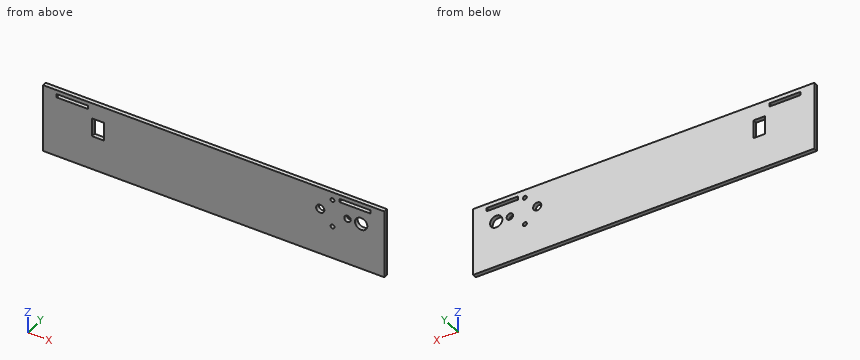
```python
from build123d import *

# Parameters (mm, degrees)
F0_W     = 250
F0_H     = 50
F1_DEPTH = 3
F2_DEPTH = 3
F3_R     = 4.5
F3_R_2   = 1.45
F3_R_3   = 2.375
F3_R_4   = 3
F3_W     = 8.5
F3_H     = 13.5
F4_DEPTH = 25


# Not quite as in the source:
# - ends of sketch curves that miss each other by under 0.0002 mm in the source are joined


with BuildPart() as f1:
    # F0 (on Front) → F1 (new body)
    with BuildSketch(Plane.XZ):
        with Locations((-42.7222467884, 16.2994446903)):
            Rectangle(F0_W, F0_H)
        Polygon((-147.7222467884, 35.7994452119), (-157.7222467884, 35.7994452119), (-157.7222467884, 38.2994446903), (-134.7222467884, 38.2994446903), (-134.7222467884, 35.7994446903), (-144.7222467884, 35.7994446903), align=None, mode=Mode.SUBTRACT)
        Polygon((49.2777532116, 38.2994446903), (62.2777532116, 38.2994446903), (72.2777532116, 38.2994446903), (72.2777532116, 35.7994446903), (49.2777532116, 35.7994446903), align=None, mode=Mode.SUBTRACT)
    extrude(amount=F1_DEPTH)

    # F0 (on Front) → F2 (join)
    with BuildSketch(Plane.XZ):
        with Locations((-42.7222467884, 16.2994446903)):
            Rectangle(F0_W, F0_H)
        Polygon((-147.7222467884, 35.7994452119), (-157.7222467884, 35.7994452119), (-157.7222467884, 38.2994446903), (-134.7222467884, 38.2994446903), (-134.7222467884, 35.7994446903), (-144.7222467884, 35.7994446903), align=None, mode=Mode.SUBTRACT)
        Polygon((49.2777532116, 38.2994446903), (62.2777532116, 38.2994446903), (72.2777532116, 38.2994446903), (72.2777532116, 35.7994446903), (49.2777532116, 35.7994446903), align=None, mode=Mode.SUBTRACT)
    extrude(amount=F2_DEPTH)

    # F3 (on face) → F4 (cut)
    with BuildSketch(Plane(origin=(0, 0, 0), x_dir=(-1, 0, 0), z_dir=(0, 1, 0))):
        with Locations((-65.2777532116, 25.2994446903)):
            Circle(F3_R)
        with Locations((-44.2777532116, 15.2994446903)):
            Circle(F3_R_2)
        with Locations((-44.2777532116, 35.2994446903)):
            Circle(F3_R_2)
        with Locations((-55.2777532116, 25.2994446903)):
            Circle(F3_R_3)
        with Locations((-35.2777532116, 25.2994446903)):
            Circle(F3_R_4)
        with Locations((127.4722467884, 23.0494446903)):
            Rectangle(F3_W, F3_H)
    extrude(amount=-F4_DEPTH, mode=Mode.SUBTRACT)


solid = f1.part
```
CAD build for the part. Positions are in the model's coordinates, mm. Give positions to 0.01 mm unless a question says otherwise; leave off trailing zeros. Write each loop counter-clockwise with the first axis right and the second up, starting at its lowest first coordinate (ties: lowest second). Pieces come first, ordered by that corner, then holes. Notation, with made-up numbers: M 25,6 L 65,6 A20 ccw 65,11 Z; hole C -26,76 d2. An arc over 180 degrees is marked long. Return JSON: item names as keys, results as strings. Group by question number.
(1) Flat gauge pin, fed straight in: pin 1 Ø2.5 at (x, z) = (44.28, 35.3) entering from +Y. Where does the tip first touch, or does it go through?
(2) Drill centre lines: L1, parallel to X at y = -1.6, z = 35; L2, parallel to Z at x = 70, y = -1.25; L3, parallel to X at y = -2.45, z = 17.5. Where is each one in solid material? Low to high. Write a range as [from, to].
(3) Band-saw the part on B-B (y = -2.4). State how many separate pieces and enclosed holes the cut face has, and give its area (3 significant figures).
(4) Band-saw the part on A-A (x = -140.5). Give the cut face in (y, z), and give its area (4 significant figures).
Entries:
{
 "1": {"pin 1": "passes through"},
 "2": {"L1": "x = [-167.72, 42.86], [45.7, 82.28]", "L2": "z = [-8.7, 35.8], [38.3, 41.3]", "L3": "x = [-167.72, -131.72], [-123.22, 82.28]"},
 "3": {"separate pieces": "1", "enclosed holes": "8", "area": "12,100 mm^2"},
 "4": {"outline": "M -3,-8.7 L 0,-8.7 L 0,35.8 L -3,35.8 Z; M -3,38.3 L 0,38.3 L 0,41.3 L -3,41.3 Z", "area": "142.5 mm^2"}
}
